Study the drawing (mm; zero at the part's minimum x, y, z) and answer. A direction names the side the tool comes from. Coordinates: 2 decimals unless noted, no trailing zeros. Loops run counter-clockwise (first coordinate to the right, second up) from the corner with the lowest first, then second, coordinate; pieces in that order, holes last. Notation, with made-up numbers: (54, 44) -> (59, 44) arc R18 cw to (59, 51) -> close; hole circle Ø5 at (-21, 53.25). An arc over 180 degrees is marked (long way). One line per question, with ' | ' between items.
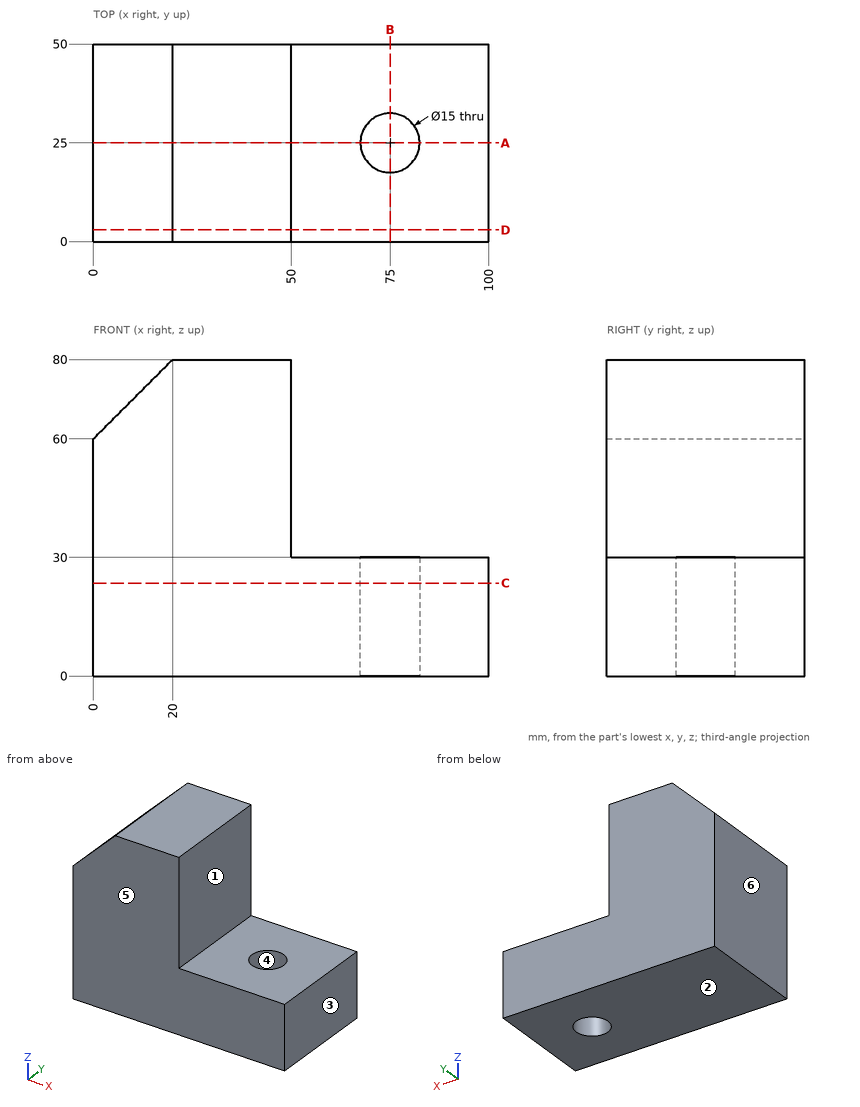
1) Find section A-A (y = 25). Write down the section's boundary in (x, z).
Check values:
outline: (0, 0) -> (67.5, 0) -> (67.5, 30) -> (50, 30) -> (50, 80) -> (20, 80) -> (0, 60) -> close; (82.5, 0) -> (100, 0) -> (100, 30) -> (82.5, 30) -> close
2) Flat-ended cylindrical pins translate along their axes: pin 1 (4 mm diameter, centred on y = 15.5, z = 68.5, fed in from +X); pin 2 (1 mm diameter, centred on x = 59.5, y = 30.5, fed in from -Z); pin 3 (17 mm diameter, centred on x = 75, y = 25, fed in from +Z). Find the tip coordinate at first contact, or state that the pin passes through.
Check values:
pin 1: stops at x = 50 | pin 2: stops at z = 0 | pin 3: stops at z = 30
3) Find section C-C (z = 23.5). Write down the section's boundary in (x, y), plus the area to 3 significant figures.
Check values:
outline: (0, 0) -> (100, 0) -> (100, 50) -> (0, 50) -> close; hole circle Ø15 at (75, 25) | area: 4,820 mm^2
4) The mould has two halves that part along X. Classify the marked faces 3, 4, 5 and 6: released by +X, released by -X, zero draft, split by the parting line, or undercut.
Check values:
face 3: released by +X | face 4: undercut | face 5: zero draft | face 6: released by -X
5) Find the intervals of material crossed by line 1 along X through (y, z) = (25.5, 24); line 2 along X through (y, z) = (27, 42); line 3 along Z through (x, y) = (90, 25.5), in increasing order.
Check values:
line 1: x = 0 to 67.52, 82.48 to 100 | line 2: x = 0 to 50 | line 3: z = 0 to 30
6) For the marked faces 1 and 2, determine the directions among +Z, -Z, +X, -X, +Y, -Y from which every point of the face is accessible in a straight line to the end or side of a thin tool.
Check values:
face 1: +Z, +X, +Y, -Y | face 2: -Z, +X, -X, +Y, -Y
7) Find section D-D (y = 3). Write down the section's boundary in (x, z).
Check values:
outline: (0, 0) -> (100, 0) -> (100, 30) -> (50, 30) -> (50, 80) -> (20, 80) -> (0, 60) -> close
8) Find section B-B (x = 75). Write down the section's boundary in (y, z), plus the area to 3 significant figures.
Check values:
outline: (0, 0) -> (17.5, 0) -> (17.5, 30) -> (0, 30) -> close; (32.5, 0) -> (50, 0) -> (50, 30) -> (32.5, 30) -> close | area: 1,050 mm^2
